The drawing under review shows one solid part. Ordinate dimensions are in mm from its lowest x, y, z. A direction names the side the tool comes from. Round coordinates to 2 decimals unless told otherwise and drop trailing zeros. Write each loop counter-clockwise with the first axis right and the second up, starting at its lowest first coordinate (ties: lowest second). Pieces come first, ordered by that corner, then holes. Notation, with made-up numbers: (-28.5, 42.25) -> (-4.5, 42.25) arc R22 ccw to (-4.5, 61.25) -> close; hole circle Ø10 at (75, 5.5). An arc over 180 degrees is marked (long way). Use CSV: the item, a comma, the result in double quotes. Start each with the question number.
1) Take a section at B-B, the plane z = 35.5. Give the boundary of the cut face in (x, y).
2) Take a section at D-D, the plane y = 49. Give the boundary of the cut face in (x, z), then the cut area to 3 significant figures.
3) Wall thickness on probe 1 along Z at (x, y) = (20, 27); probe 2 along Z at (x, y) = (108.5, 21); probe 3 along Y at (x, z) = (63, 40.5): over which ranges is each line inside the solid? List them lowest first. Write a range as [from, to].
4) Take a section at C-C, the plane x = 74. Give the boundary of the cut face in (y, z).
5) For pin 1 Ø21 at (x, y) = (105.5, 40) entering from +Z; pin 2 Ø5 at (x, z) = (19, 30) entering from -Y; pin 3 Ø6.5 at (x, y) = (66.5, 7) entering from +Z, all flat-tipped, find the tip position at first contact; note any pin that passes through.
6) Machinability: for the marked faces 1, 2 and 3, which of the approach directions +Z, -Z, +X, -X, +Y, -Y give a long, thin tool a straight path to every point of the face, cutting with its end or side? Answer none if there is none.
7) Take a section at A-A, the plane y = 17.5. Give the boundary of the cut face in (x, z).
8) Mouldability with a two-part tool opening along X and no side actions: class the marked faces 4, 5, 6 and 7 as released by +X, released by -X, zero draft, split by the parting line, or undercut.
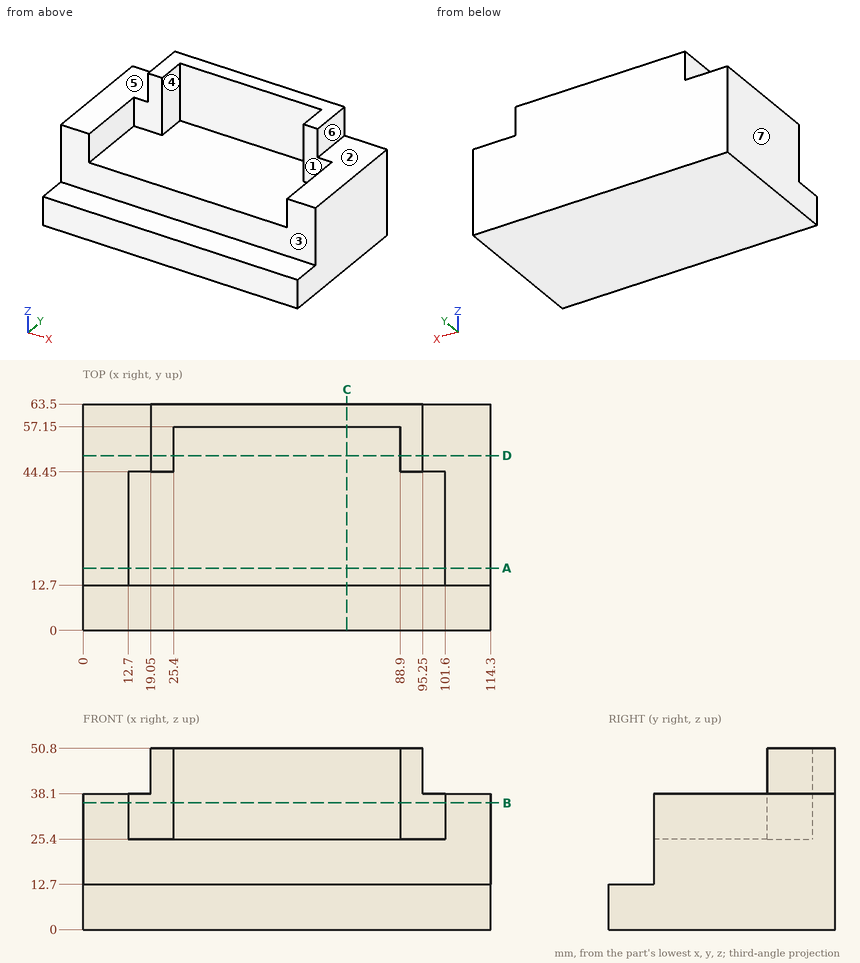
Values found:
1,outline,"(0, 12.7) -> (12.7, 12.7) -> (12.7, 44.45) -> (25.4, 44.45) -> (25.4, 57.15) -> (88.9, 57.15) -> (88.9, 44.45) -> (101.6, 44.45) -> (101.6, 12.7) -> (114.3, 12.7) -> (114.3, 63.5) -> (0, 63.5) -> close"
2,outline,"(0, 0) -> (114.3, 0) -> (114.3, 38.1) -> (95.25, 38.1) -> (95.25, 50.8) -> (88.9, 50.8) -> (88.9, 25.4) -> (25.4, 25.4) -> (25.4, 50.8) -> (19.05, 50.8) -> (19.05, 38.1) -> (0, 38.1) -> close"
2,area,"3,710 mm²"
3,probe 1,"[0, 25.4]"
3,probe 2,"[0, 38.1]"
3,probe 3,"[57.15, 63.5]"
4,outline,"(0, 0) -> (63.5, 0) -> (63.5, 50.8) -> (57.15, 50.8) -> (57.15, 25.4) -> (12.7, 25.4) -> (12.7, 12.7) -> (0, 12.7) -> close"
5,pin 1,"z = 38.1"
5,pin 2,"y = 44.45"
5,pin 3,"z = 12.7"
6,face 1,"+Z, -Y"
6,face 2,"+Z, +X, +Y, -Y"
6,face 3,"+Z, +X, -X, -Y"
7,outline,"(0, 0) -> (114.3, 0) -> (114.3, 38.1) -> (101.6, 38.1) -> (101.6, 25.4) -> (12.7, 25.4) -> (12.7, 38.1) -> (0, 38.1) -> close"
8,face 4,"undercut"
8,face 5,"zero draft"
8,face 6,"released by +X"
8,face 7,"released by -X"
